from build123d import *

# Parameters (mm, degrees)
SKETCH_1_W           = 20
SKETCH_1_H           = 28
SKETCH_1_R           = 1.6
EXTRUDE_1_DEPTH      = 5
EXTRUDE_2_DEPTH      = 5
EXTRUDE_2_DEPTH_BACK = 1.1
SKETCH_3_W           = 6.1
SKETCH_3_H           = 30.125226912
EXTRUDE_3_DEPTH      = 7
SKETCH_4_R           = 1.35
CUT_EXTRUDE_1_DEPTH  = 7
SKETCH_5_W           = 5
SKETCH_5_H           = 28
CUT_EXTRUDE_2_DEPTH  = 10
CUT_EXTRUDE_3_DEPTH  = 10


with BuildPart() as part:
    # 草图1 → 凸台-拉伸1 (new body)
    with BuildSketch(Plane(origin=(0, 0, 0), x_dir=(1, 0, 0), z_dir=(0, 1, 0))):
        Rectangle(SKETCH_1_W, SKETCH_1_H)
        with Locations(Location((-5, 10, 0), (0, 0, 270))):
            Circle(SKETCH_1_R, mode=Mode.SUBTRACT)
        with Locations(Location((5, 10, 0), (0, 0, 90))):
            Circle(SKETCH_1_R, mode=Mode.SUBTRACT)
        with Locations(Location((5, -10, 0), (0, 0, 270))):
            Circle(SKETCH_1_R, mode=Mode.SUBTRACT)
        with Locations(Location((-5, -10, 0), (0, 0, 90))):
            Circle(SKETCH_1_R, mode=Mode.SUBTRACT)
    extrude(amount=EXTRUDE_1_DEPTH)

    # 草图2 → 凸台-拉伸2 (add, two sides: drawn at the far end of the back side and taken through both)
    with BuildSketch(Plane(origin=(0, 0, 0), x_dir=(0, 0, -1), z_dir=(1, 0, 0)).offset(-EXTRUDE_2_DEPTH_BACK)):
        with BuildLine():
            Line((42.482395746, 143.5), (42.482395746, 113.374773088))
            add(Edge.make_bspline(
                [(10.794309538, 5), (-3.625508376, 21.700163207), (-0.038874902, 68.530494039), (24.786643579, 102.563540472), (42.482395746, 113.374773088)],
                knots=[0, 0, 0, 0, 0.510479212, 1, 1, 1, 1], degree=3))
            Line((10.794309538, 5), (-14, 5))
            add(Edge.make_bspline(
                [(-14, 5), (-21.090980053, 28.072383436), (-16.059602837, 83.599622922), (19.318940175, 126.307389699), (42.482395746, 143.5)],
                knots=[0, 0, 0, 0, 0.452386754, 1, 1, 1, 1], degree=3))
        make_face()
    extrude(amount=EXTRUDE_2_DEPTH + EXTRUDE_2_DEPTH_BACK)

    # 草图3 → 凸台-拉伸3 (add)
    with BuildSketch(Plane(origin=(0, 0, -42.482395746), x_dir=(-1, 0, 0), z_dir=(0, 0, -1))):
        with Locations((-1.95, 128.437386544)):
            Rectangle(SKETCH_3_W, SKETCH_3_H)
    extrude(amount=EXTRUDE_3_DEPTH)

    # 草图4 → 切除-拉伸1 (cut)
    with BuildSketch(Plane(origin=(5, 0, 0), x_dir=(0, 0, -1), z_dir=(1, 0, 0))):
        with Locations((45.982395746, 136.5)):
            Circle(SKETCH_4_R)
        with Locations((45.982395746, 121.5)):
            Circle(SKETCH_4_R)
    extrude(amount=-CUT_EXTRUDE_1_DEPTH, mode=Mode.SUBTRACT)


with BuildPart() as body_2:
    # 镜向1: mirrored copy
    add(part.part.mirror(Plane(origin=(20, 0, 0), x_dir=(0, 0, 1), z_dir=(1, 0, 0))))

    # 草图5 → 切除-拉伸2 (cut)
    with BuildSketch(Plane(origin=(0, 5, 0), x_dir=(1, 0, 0), z_dir=(0, 1, 0))):
        with Locations((32.5, 0)):
            Rectangle(SKETCH_5_W, SKETCH_5_H)
    extrude(amount=-CUT_EXTRUDE_2_DEPTH, mode=Mode.SUBTRACT)

    # 草图6 → 切除-拉伸3 (cut)
    with BuildSketch(Plane(origin=(41.1, 0, 0), x_dir=(0, 0, -1), z_dir=(1, 0, 0))):
        with BuildLine():
            Line((47.182395746, 141.5), (47.182395746, 121.5))
            ThreePointArc((47.182395746, 121.5), (45.982395746, 120.3), (44.782395746, 121.5))
            Line((44.782395746, 121.5), (44.782395746, 141.5))
            ThreePointArc((44.782395746, 141.5), (45.982395746, 142.7), (47.182395746, 141.5))
        make_face()
    extrude(amount=-CUT_EXTRUDE_3_DEPTH, mode=Mode.SUBTRACT)


solid = body_2.part
Part model, mm, in its own coordinate system. A direction names the side the tool comes from. Coordinates: 2 decimals unless noted, no trailing zeros. Loops run counter-clockwise (first coordinate to the right, second up) from the corner with the lowest first, then second, coordinate; pieces in that order, holes last. Notation, with made-up numbers: (5, -28.75) -> (37, -28.75) arc R10 cw to (37, -15.75) -> close; hole circle Ø8 at (72, 23). An arc over 180 degrees is marked (long way). Use a Markdown table: item, result. Add a question column.
Item 1: Which spindle directions (+Z, -Z, +X, -X, +Y, -Y) get a long thin tool onto all of the face, cutting with end or side? Do faces 4 (the flat face through (38, 129, -44.782)), 5 (the flat face through (43, 2, -14)), 6 (the flat face through (35, 3, -13)), 7 (the cylindrical face through (36.6, 2.5, 10)). Say none if no direction does.
Item 2: Band-saw the part on A-A on x = 48.5. Write the cut outline in (y, z).
Item 3: Flat gauge pins, fed straight in: P1, Ø5, axis at x = 38.5, y = 139, coming from the +Z side; P2, Ø7.5, axis at x = 39.5, z = 4.5, coming from the +Y side; P3, Ø0.5, axis at x = 36, z = 10, coming from the -Y side. Where does each tip first touch, or does it go through?
Item 4: Probe probe 1 along X at (y, z) = (3.05, 10); probe 2 along Y at (x, z) = (41.5, 1); probe 3 along X at (y, z) = (120.5, -42). List the from-to ranges inside material, lowest first.
Item 5: Pull direction Z, two halves, no side cores. Call faces 1 (the flat face through (43, 2, 14)), 2 (the flat face through (41.1, 79, -6)), 3 (the cylindrical face through (38.1, 142.7, -46)): +Z half, -Z half, draft (parallel to the pull), parting line (faces both ways), or undercut.
Geometry says:
| question | item | result |
|---|---|---|
| 1 | face 4 | +X, -X |
| 1 | face 5 | -Z, +X, -X, -Y |
| 1 | face 6 | +Z, -Z, -X, +Y, -Y |
| 1 | face 7 | -X, -Y |
| 2 | outline | (0, -14) -> (5, -14) -> (5, 14) -> (0, 14) -> close |
| 3 | P1 | z = -33.67 |
| 3 | P2 | y = 95.79 |
| 3 | P3 | y = 5 |
| 4 | probe 1 | 36.6 to 43.4, 46.6 to 50 |
| 4 | probe 2 | 0 to 5 |
| 4 | probe 3 | 35 to 41.1 |
| 5 | face 1 | +Z half |
| 5 | face 2 | draft |
| 5 | face 3 | undercut |
